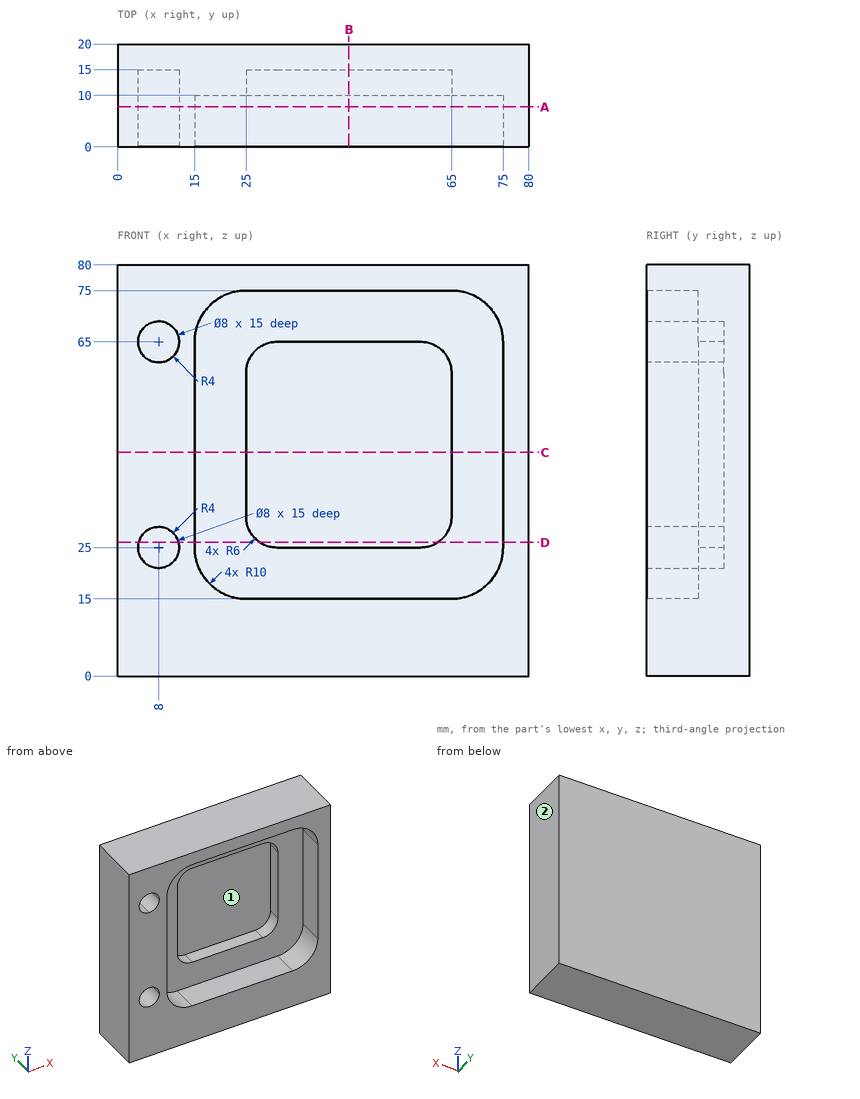
For this review, use the dimensioned drawing (mm, ordinates from the lowest corner) and the shaded views. A direction names the side the tool comes from. Round coordinates to 2 decimals unless told otherwise and drop trailing zeros. Order: outer loops, then holes, each group sorted by start corner. A loop starts at its lowest first (then second) coordinate and runs counter-clockwise, first axis right, second up. Notation, with made-up numbers: M 31.5,21 L 48.5,21 A16 ccw 48.5,51 Z; hole C -25,11.5 d6. An arc over 180 degrees is marked long. Use a Markdown table: item, result. Add a question column.
Item 1: Insertion check: pin 1 (8 mm diameter, centred on x = 59, z = 38, fed in from -Y). The pin has a flat end and moves straight along its axis. Give the tip position at first contact, or say it passes through.
Item 2: Add section D-D, the plane z = 26. Give the boundary of the cut face in (x, y).
Item 3: Add section A-A, the plane y = 7.75. Give the boundary of the cut face in (x, z), then the cut area to 3 significant figures.
Item 4: Tool access review of the marked faces 1 and 2: name each direction out of +Z, -Z, +X, -X, +Y, -Y from which nothing blocks a thin tool from reaching the whole face with its end or side.
Item 5: To check wall thickness, follow line 1 along Z through (x, y) = (8, 8.75); line 2 along X through (y, z) = (6, 25); line 3 along X through (y, z) = (6.5, 59). State the ranges of each line that lie inside material, in increasing order.
Item 6: Add section B-B, the plane x = 45. Give the boundary of the cut face in (y, z), then the cut area to 3 significant figures.
Item 7: Add section C-C, the plane z = 43.5. Give the boundary of the cut face in (x, y), then the cut area to 3 significant figures.
Geometry results:
| question | item | result |
|---|---|---|
| 1 | pin 1 | stops at y = 15 |
| 2 | outline | M 0,0 L 4.13,0 L 4.13,15 L 11.87,15 L 11.87,0 L 15,0 L 15,10 L 27.68,10 L 27.68,15 L 62.32,15 L 62.32,10 L 75,10 L 75,0 L 80,0 L 80,20 L 0,20 Z |
| 3 | outline | M 0,0 L 80,0 L 80,80 L 0,80 Z; hole C 8,25 d8; hole C 8,65 d8; hole M 15,25 A10 ccw 25,15 L 65,15 A10 ccw 75,25 L 75,65 A10 ccw 65,75 L 25,75 A10 ccw 15,65 Z |
| 3 | area | 2,790 mm² |
| 4 | face 1 | -Y |
| 4 | face 2 | +Z, -Z, +X, +Y, -Y |
| 5 | line 1 | z = 0 to 21, 29 to 61, 69 to 80 |
| 5 | line 2 | x = 0 to 4, 12 to 15, 75 to 80 |
| 5 | line 3 | x = 0 to 15, 75 to 80 |
| 6 | outline | M 0,0 L 20,0 L 20,80 L 0,80 L 0,75 L 10,75 L 10,65 L 15,65 L 15,25 L 10,25 L 10,15 L 0,15 Z |
| 6 | area | 800 mm² |
| 7 | outline | M 0,0 L 15,0 L 15,10 L 25,10 L 25,15 L 65,15 L 65,10 L 75,10 L 75,0 L 80,0 L 80,20 L 0,20 Z |
| 7 | area | 800 mm² |
